Part print with two shaded views. Sizes in mm from the minimum x, y, z corner. A direction names the side the tool comes from. Round coordinates to 2 decimals unless told otherwise and drop trailing zeros. Write each loop counter-clockwise with the first axis right and the second up, starting at its lowest first coordinate (ties: lowest second). Pieces come first, ordered by that corner, then holes. Notation, with made-up numbers: (57, 84.25) - (90, 84.25) arc R20 cw to (90, 91.25) - close; hole circle Ø7 at (40, -24). An arc over 180 degrees is marked (long way). Answer as a JSON object with one key per item and string values. Group by question number.
Item 1: Which spindle directions (+Z, -Z, +X, -X, +Y, -Y) get a long thin tool onto all of the face, cutting with end or side? Do the marked faces 1, 2 and 3. Say none if no direction does.
Item 2: Probe line 1 (Z direction, x = 12, y = 15); line 2 (X direction, y = 27, z = 11); line 3 (Y direction, x = 18.5, z = 35.5). List the from-to ranges inside material, lowest first. Write a range as from..to.
Item 3: Slice it at B-B, the plane x = 8. List the corners of the cut face in (y, z), then the cut area to 3 significant figures.
Item 4: Slice it at A-A, the plane y = 35. List the corners of the cut face in (x, z).
Item 5: Flat gauge pins, fed straight in: pin 1 (5 mm diameter, centred on x = 19.5, z = 27.5, fed in from +Y); pin 2 (10 mm diameter, centred on x = 16, y = 15, fed in from -Z); pin 3 (12 mm diameter, centred on x = 17.5, z = 36, fed in from -Y). Where does each tip first touch, or does it go through?
Item 6: Slice it at C-C, the plane z = 58. List the corners of the cut face in (x, y).
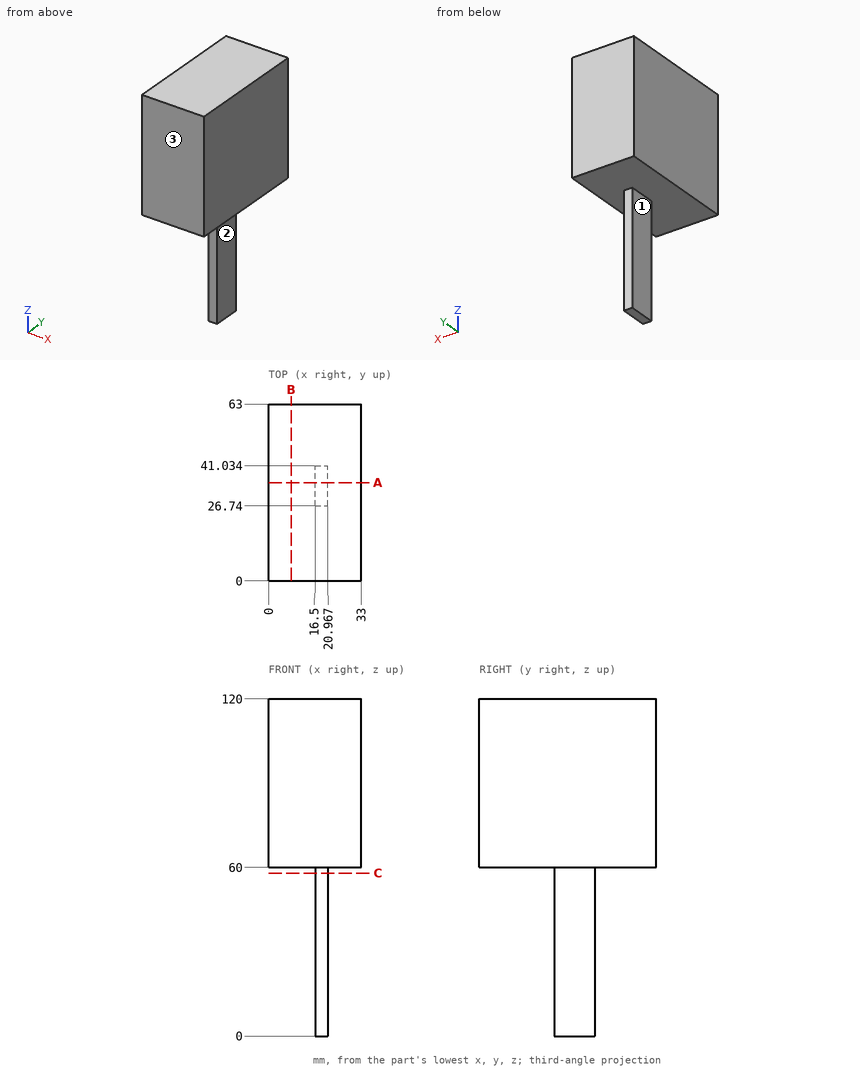
Geometry says:
{
 "1": {"face 1": "-Z, -X, +Y, -Y", "face 2": "-Z, +X, +Y, -Y", "face 3": "+Z, -Z, +X, -X, -Y"},
 "2": {"line 1": "z = 60..120", "line 2": "x = 16.5..20.97", "line 3": "y = 26.74..41.03"},
 "3": {"outline": "(0, 60) - (63, 60) - (63, 120) - (0, 120) - close", "area": "3,780 mm^2"},
 "4": {"outline": "(0, 60) - (16.5, 60) - (16.5, 0) - (20.97, 0) - (20.97, 60) - (33, 60) - (33, 120) - (0, 120) - close"},
 "5": {"pin 1": "stops at y = 41.03", "pin 2": "stops at z = 60", "pin 3": "stops at y = 26.74"},
 "6": {"outline": "(16.5, 26.74) - (20.97, 26.74) - (20.97, 41.03) - (16.5, 41.03) - close"}
}
